Geometry: final body of the model. Coordinates: model frame, mm. A direction names the side the tool comes from. Give positions to 0.01 mm unless a question says otherwise; leave off trailing zeros. Write each loop counter-clockwise with the first axis right and the second up, starting at its lowest first coordinate (ties: lowest second). Pieces come first, ordered by that corner, then holes.
Q1. Section B-B (x = -29.5). Return the cut outline in (y, z).
Q2. Section C-C (z = -16). Return the cut outline in (x, y), plus the area to 3 significant figures.
Q3. Section A-A (x = 15.5). Return the cut outline in (y, z).
Q4. Reachability of faces 5 (the cylindrical face through (40.022, 1.232, 14.734)), 6 (the cylindrical face through (-37.88, 3.77, -10.53)) from +Z, -Z, +X, -X, +Y, -Y: full face, straight path, thin tool, end or side. Return the list, or none.
Q5. Pin query (flat end, axial travel): pin 1 Ø4 at (x, z) = (-40.5, -9.7) entering from +Y; pin 2 Ø2.5 at (x, z) = (-41.5, 11.7) entering from +Y; pin 3 Ø2 at (x, y) = (10.5, 3.5) entering from -Z. Return the tip coordinate at first contact, or that it passes through.
Q6. Line query: line 1 (X direction, y = 1.5, z = 15.2); line 2 (X direction, y = 1.3, z = -9.7); line 3 (Z direction, x = -40.5, y = 3.6). Output: solid intervals per line, ascending.
Q7. Mould query, pull axis Z, two halves, no side actions, for faces 1 (the cylindrical face through (43.6, 1.01, 17.34)), 2 (the flat face through (42.3, 2.5, -9.7)), 3 (the flat face through (17, 2.5, 16)), 4 (the flat face through (-1, 0, 0)). Classes: +Z half, -Z half, draft (parallel to the pull), parting line (faces both ways), or undercut.
from build123d import *

# Parameters (mm, degrees)
SKETCH1_W                        = 89
SKETCH1_H                        = 36.4
BOSS_EXTRUDE1_DEPTH              = 5
CBORE_FOR_M2_5_SHCS1_D           = 3.1
CBORE_FOR_M2_5_SHCS1_CBORE_D     = 5.5
CBORE_FOR_M2_5_SHCS1_CBORE_DEPTH = 2.5
FILLET3_R                        = 3
FILLET4_R                        = 3


with BuildPart() as part:
    # Sketch1 → Boss-Extrude1 (new body)
    with BuildSketch(Plane(origin=(0, 0, 0), x_dir=(1, 0, 0), z_dir=(0, 1, 0))):
        Rectangle(SKETCH1_W, SKETCH1_H)
    extrude(amount=BOSS_EXTRUDE1_DEPTH)

    # CBORE for M2.5 SHCS1 (through all)
    with Locations(Plane(origin=(0, 5, 0), x_dir=(1, 0, 0), z_dir=(0, 1, 0))):
        with Locations((-40.5, 9.7), (-41.5, -11.7), (15.5, -15.2), (41.5, -15.2), (40.5, 9.7)):
            CounterBoreHole(CBORE_FOR_M2_5_SHCS1_D / 2, CBORE_FOR_M2_5_SHCS1_CBORE_D / 2, CBORE_FOR_M2_5_SHCS1_CBORE_DEPTH)

    # Fillet3
    fillet3_edges = [part.edges().sort_by_distance(p)[0] for p in [
        (44.5, 2.5, 18.2),
        (-44.5, 2.5, 18.2),
        (-44.5, 2.5, -18.2),
        (44.5, 2.5, -18.2),
    ]]
    fillet(fillet3_edges, radius=FILLET3_R)

    # Fillet4
    # the kernel refuses this fillet: 3 mm, written as the material it takes off along each edge
    with BuildSketch(Plane(origin=(-41.5, 5, -15.2), x_dir=(-1, 0, 0), z_dir=(0, 0, 1))) as fillet4_piece_1:
        with BuildLine():
            CenterArc((3 - FILLET4_R, FILLET4_R), FILLET4_R, 270, 90)
            Line((3, FILLET4_R), (3, 0))
            Line((3, 0), (3 - FILLET4_R, 0))
        make_face()
    revolve(axis=Axis((-41.5, 5, -15.2), (0, -1, 0)), revolution_arc=90, mode=Mode.SUBTRACT)
    with BuildSketch(Plane(origin=(41.5, 5, -18.2), x_dir=(0, 0, 1), z_dir=(-1, 0, 0))) as fillet4_piece_2:
        with BuildLine():
            CenterArc((FILLET4_R, -FILLET4_R), FILLET4_R, 90, 90)
            Line((0, -FILLET4_R), (0, 0))
            Line((0, 0), (FILLET4_R, 0))
        make_face()
    extrude(amount=83, mode=Mode.SUBTRACT)
    with BuildSketch(Plane(origin=(41.5, 5, -15.2), x_dir=(1, 0, 0), z_dir=(0, 0, 1))) as fillet4_piece_3:
        with BuildLine():
            CenterArc((3 - FILLET4_R, -FILLET4_R), FILLET4_R, 0, 90)
            Line((3, -FILLET4_R), (3, 0))
            Line((3, 0), (3 - FILLET4_R, 0))
        make_face()
    revolve(axis=Axis((41.5, 5, -15.2), (0, 1, 0)), revolution_arc=90, mode=Mode.SUBTRACT)
    with BuildSketch(Plane(origin=(44.5, 5, 15.2), x_dir=(-1, 0, 0), z_dir=(0, 0, -1)), Plane(origin=(-44.5, 5, -15.2), x_dir=(1, 0, 0), z_dir=(0, 0, 1))) as fillet4_piece_4:
        with BuildLine():
            CenterArc((FILLET4_R, -FILLET4_R), FILLET4_R, 90, 90)
            Line((0, -FILLET4_R), (0, 0))
            Line((0, 0), (FILLET4_R, 0))
        make_face()
    extrude(amount=30.4, mode=Mode.SUBTRACT)
    with BuildSketch(Plane(origin=(-41.5, 5, 18.2), x_dir=(0, -1, 0), z_dir=(1, 0, 0))) as fillet4_piece_5:
        with BuildLine():
            CenterArc((FILLET4_R, FILLET4_R), FILLET4_R, 180, 90)
            Line((0, FILLET4_R), (0, 0))
            Line((0, 0), (FILLET4_R, 0))
        make_face()
    extrude(amount=83, mode=Mode.SUBTRACT)
    with BuildSketch(Plane(origin=(-41.5, 5, 15.2), x_dir=(0, 0, 1), z_dir=(1, 0, 0))) as fillet4_piece_6:
        with BuildLine():
            CenterArc((3 - FILLET4_R, FILLET4_R), FILLET4_R, 270, 90)
            Line((3 - FILLET4_R, 0), (3, 0))
            Line((3, 0), (3, FILLET4_R))
        make_face()
    revolve(axis=Axis((-41.5, 5, 15.2), (0, -1, 0)), revolution_arc=90, mode=Mode.SUBTRACT)
    with BuildSketch(Plane(origin=(41.5, 5, 15.2), x_dir=(0, 0, 1), z_dir=(-1, 0, 0))) as fillet4_piece_7:
        with BuildLine():
            CenterArc((3 - FILLET4_R, -FILLET4_R), FILLET4_R, 0, 90)
            Line((3 - FILLET4_R, 0), (3, 0))
            Line((3, 0), (3, -FILLET4_R))
        make_face()
    revolve(axis=Axis((41.5, 5, 15.2), (0, 1, 0)), revolution_arc=90, mode=Mode.SUBTRACT)


solid = part.part
Computed:
1. outline: (0, -18.2) - (2, -18.2) arc R3 ccw to (5, -15.2) - (5, 15.2) arc R3 ccw to (2, 18.2) - (0, 18.2) - close
2. outline: (-44.39, 0) - (44.39, 0) - (44.39, 2) arc R2.89 ccw to (41.5, 4.89) - (-41.5, 4.89) arc R2.89 ccw to (-44.39, 2) - close
2. area: 431 mm2
3. outline: (0, -18.2) - (2, -18.2) arc R3 ccw to (5, -15.2) - (5, 12.45) - (2.5, 12.45) - (2.5, 13.65) - (0, 13.65) - close; (0, 16.75) - (2.5, 16.75) - (2.5, 17.95) - (3.2, 17.95) arc R3 ccw to (2, 18.2) - (0, 18.2) - close
4. face 5: +Y, -Y
4. face 6: +Y
5. pin 1: stops at y = 2.5
5. pin 2: passes through
5. pin 3: stops at z = -18.16
6. line 1: x = -44.5 to 13.95, 17.05 to 39.95, 43.05 to 44.5
6. line 2: x = -44.5 to -42.05, -38.95 to 38.95, 42.05 to 44.5
6. line 3: z = -17.74 to -12.45, -6.95 to 9.14, 14.26 to 17.74
7. face 1: +Z half
7. face 2: undercut
7. face 3: undercut
7. face 4: draft
